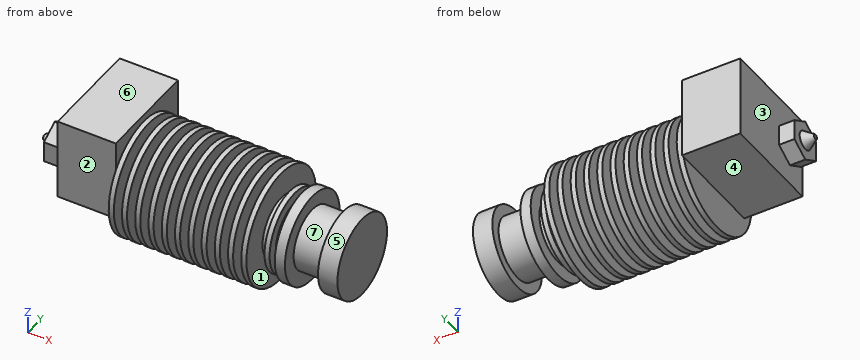
```python
from build123d import *

# Parameters (mm, degrees)
SKETCH_3_R      = 3.5
EXTRUDE_1_DEPTH = 3
SKETCH_4_W      = 16
SKETCH_4_H      = 20
EXTRUDE_2_DEPTH = 11.4
EXTRUDE_3_DEPTH = 3
SKETCH_6_R      = 1.8
SKETCH_7_R      = 0.5


with BuildPart() as part:
    # 草圖1 → 旋轉1 (revolve)
    with BuildSketch(Plane.XY, mode=Mode.PRIVATE) as revolve_1_sk:
        Polygon((-26, 0), (-26, 11.2), (-25, 11.2), (-25, 6), (-23.4, 6), (-23.4, 11.2), (-22.4, 11.2), (-22.4, 6), (-20.8, 6), (-20.8, 11.2), (-19.8, 11.2), (-19.8, 6), (-18.2, 6), (-18.2, 11.2), (-17.2, 11.2), (-17.2, 6), (-15.6, 6), (-15.6, 11.2), (-14.6, 11.2), (-14.6, 6), (-13, 6), (-13, 11.2), (-12, 11.2), (-12, 6), (-10.4, 6), (-10.4, 11.2), (-9.4, 11.2), (-9.4, 6), (-7.8, 6), (-7.8, 11.2), (-6.8, 11.2), (-6.8, 6), (-5.2, 6), (-5.2, 11.2), (-4.2, 11.2), (-4.2, 6), (-2.6, 6), (-2.6, 11.2), (-1.6, 11.2), (-1.6, 6), (0, 6), (0, 11.2), (1, 11.2), (1, 6), (2.6, 6), (2.6, 0), (1, 0), (0, 0), align=None)
    revolve(revolve_1_sk.sketch.rotate(Axis((0, 0, 0), (-1, 0, 0)), 90), axis=Axis((0, 0, 0), (-1, 0, 0)))

    # 草圖2 → 旋轉2 (revolve)
    with BuildSketch(Plane.XY):
        Polygon((2.6, 0), (2.6, 8), (3.6, 8), (3.6, 6), (5.1, 6), (5.1, 8.79813536), (7.1, 8.79813536), (7.1, 6), (13.1, 6), (13.1, 8), (16.9, 8), (16.9, 0), align=None)
    revolve(axis=Axis((16.9, 0, 0), (-1, 0, 0)))

    # 草圖3 → 填料-伸長1 (add)
    with BuildSketch(Plane.ZY.offset(26)):
        Circle(SKETCH_3_R)
    extrude(amount=EXTRUDE_1_DEPTH)

    # 草圖4 → 填料-伸長2 (add)
    with BuildSketch(Plane.ZY.offset(29)):
        with Locations((0, 6)):
            Rectangle(SKETCH_4_W, SKETCH_4_H)
    extrude(amount=EXTRUDE_2_DEPTH)

    # 草圖5 → 填料-伸長3 (add)
    with BuildSketch(Plane.ZY.offset(40.4)):
        Polygon((4.041451884, 0), (2.020725942, 3.5), (-2.020725942, 3.5), (-4.041451884, 0), (-2.020725942, -3.5), (2.020725942, -3.5), align=None)
    extrude(amount=EXTRUDE_3_DEPTH)

    # 草圖6 → 疊層拉伸1 section 0
    with BuildSketch(Plane.ZY.offset(43.4)):
        Circle(SKETCH_6_R)
    # 草圖7 → 疊層拉伸1 section 1
    with BuildSketch(Plane.ZY.offset(45.4)):
        Circle(SKETCH_7_R)
    loft()


solid = part.part
```
Source: CAD feature listing. Evaluate the final solid. Frame: model axes, mm. Face numbers are marked on the shaded views. A direction names the side the tool comes from. Give positions to 0.01 mm unless a question says otherwise; leave off trailing zeros. Loops run counter-clockwise (first coordinate to the right, second up) from the corner with the lowest first, then second, coordinate; pieces in that order, holes last. Notation, with made-up numbers: (69, 50.25) -> (105, 50.25) arc R20 ccw to (105, 80.25) -> close; hole circle Ø1 at (-25.75, -6). An arc over 180 degrees is marked (long way). Use a Markdown table: item, result. Add a question column.
(1) Access query for the marked faces 4, 5, 6 and 7. Directions: +Z, -Z, +X, -X, +Y, -Y. A direction counts if a zero-diameter tool reaches every point of the face in a straight line with its end or side. Return the directions, or none.
(2) Ray query, line 1 (X direction, y = 4.5, z = -2.75); line 2 (Y direction, x = -34.5, z = 7); line 3 (X direction, y = 0, z = 2). Return the intervals inside material, ascending.
(3) Pull-direction query (X, two-part tool) for the marked faces 1, 2 and 3; classes: +X half, -X half, draft (parallel to the pull), parting line (faces both ways), or undercut.
(4) Section query A-A (x = -41.5). Output: boundary loops of the cut face in (y, z), then the cut area to 3 significant figures.
(5) First-contact query: pin 1 Ø8 at (x, z) = (3.5, -0.5) entering from +Y; pin 2 Ø8 at (x, y) = (2.5, 8.5) entering from +Z; pin 3 Ø12 at (x, z) = (-1.5, 9) entering from -Y; pin 4 Ø2 at (x, y) = (-22, 12.5) entering from +Z. Flat tips, straight axial feed; report the tip coordinate or a pass-through.
(6) Section query B-B (x = -3.5). Output: boundary loops of the cut face in (y, z), then the cut area to 3 significant figures.
Checked values:
| question | item | result |
|---|---|---|
| 1 | face 4 | -Z, -X, +Y, -Y |
| 1 | face 5 | +X |
| 1 | face 6 | +Z, -X, +Y, -Y |
| 1 | face 7 | none |
| 2 | line 1 | -40.4 to -29, -26 to 16.9 |
| 2 | line 2 | -4 to 16 |
| 2 | line 3 | -43.4 to 16.9 |
| 3 | face 1 | undercut |
| 3 | face 2 | draft |
| 3 | face 3 | -X half |
| 4 | outline | (-3.5, -2.02) -> (0, -4.04) -> (3.5, -2.02) -> (3.5, 2.02) -> (0, 4.04) -> (-3.5, 2.02) -> close |
| 4 | area | 42.4 mm^2 |
| 5 | pin 1 | y = 11.2 |
| 5 | pin 2 | z = 10.12 |
| 5 | pin 3 | y = -10.79 |
| 5 | pin 4 | through |
| 6 | outline | circle Ø12 at (0, 0) |
| 6 | area | 113 mm^2 |
